Verification items for the finished model (mm, model axes). A direction names the side the tool comes from. Round coordinates to 2 decimals unless told otherwise and drop trailing zeros. Order: outer loops, then holes, each group sorted by start corner. A loop starts at its lowest first (then second) coordinate and runs counter-clockwise, first axis right, second up. Notation, with made-up numbers: (-29.75, 2.5) -> (28.25, 2.5) arc R15 ccw to (28.25, 19.5) -> close; hole circle Ø3 at (18.5, 4). An arc over 180 degrees is marked (long way). Put each result on its own line as item: value.
```python
from build123d import *
from build123d.topology import SkipClean

# Parameters (mm, degrees)
SKETCH1_R                = 20
SKETCH1_R_2              = 15
BOSS_EXTRUDE1_DEPTH      = 380
SKETCH8_R                = 20
BOSS_EXTRUDE3_DEPTH      = 60
CUT_EXTRUDE2_START       = -899.5
SKETCH9_R                = 15
CUT_EXTRUDE2_DEPTH       = 899.5
CUT_EXTRUDE16_DEPTH      = 240
CUT_EXTRUDE17_DEPTH      = 20
CUT_EXTRUDE17_DEPTH_BACK = 20
CUT_EXTRUDE19_DEPTH      = 10
CUT_EXTRUDE19_DEPTH_BACK = 10
SKETCH26_R               = 10
CUT_EXTRUDE20_DEPTH      = 30
CUT_EXTRUDE20_DEPTH_BACK = 20
SKETCH27_R               = 3.4


with BuildPart() as part:
    # Sketch1 → Boss-Extrude1 (new, symmetric)
    with BuildSketch(Plane(origin=(0, 0, 0), x_dir=(1, 0, 0), z_dir=(0, 1, 0))):
        with Locations(Location((0, 0, 0), (0, 0, 270))):
            Circle(SKETCH1_R)
        with Locations(Location((0, 0, 0), (0, 0, 270))):
            Circle(SKETCH1_R_2, mode=Mode.SUBTRACT)
    extrude(amount=BOSS_EXTRUDE1_DEPTH, both=True)

    # Sketch8 → Boss-Extrude3 (add)
    with SkipClean():  # the faces are left unmerged after this step: merging them gives an invalid solid
        with BuildSketch(Plane.XZ.offset(380)):
            with Locations(Location((0, 0, 0), (0, 0, 270))):
                Circle(SKETCH8_R)
        extrude(amount=BOSS_EXTRUDE3_DEPTH)

    # Sketch9 → Cut-Extrude2 (cut)
    with SkipClean():  # the faces are left unmerged after this step: merging them gives an invalid solid
        with BuildSketch(Plane(origin=(-32.302786122, 416.289190775, -45.221901395), x_dir=(-0.9768887275019512, 0, 0.2137484832217963), z_dir=(0, 1, 0)).offset(CUT_EXTRUDE2_START)):
            with Locations(Location((-21.890114798, 51.081437247, 0), (0, 0, 257.657886074))):
                Circle(SKETCH9_R)
        extrude(amount=CUT_EXTRUDE2_DEPTH, mode=Mode.SUBTRACT)

    # Sketch23 → Cut-Extrude16 (cut)
    with SkipClean():  # the faces are left unmerged after this step: merging them gives an invalid solid
        with BuildSketch(Plane(origin=(0, 380, 0), x_dir=(1, 0, 0), z_dir=(0, 1, 0))):
            with BuildLine():
                Line((-7, 18.734993995), (7, 18.734993995))
                ThreePointArc((7, 18.734993995), (0, 20), (-7, 18.734993995))
            make_face()
        cut_extrude16 = extrude(amount=-CUT_EXTRUDE16_DEPTH, mode=Mode.SUBTRACT)

    # Mirror1: Cut-Extrude16 across plane
    with SkipClean():  # the faces are left unmerged after this step: merging them gives an invalid solid
        add(cut_extrude16.mirror(Plane.XY), mode=Mode.SUBTRACT)

    # Sketch24 → Cut-Extrude17 (cut, two sides: drawn at the far end of the back side and taken through both)
    with SkipClean():  # the faces are left unmerged after this step: merging them gives an invalid solid
        with BuildSketch(Plane(origin=(0, 0, 0), x_dir=(0, 0, -1), z_dir=(1, 0, 0)).offset(-CUT_EXTRUDE17_DEPTH_BACK)):
            with BuildLine():
                Line((-0.5, 200), (0.5, 200))
                ThreePointArc((0.5, 200), (2.621320344, 199.121320344), (3.5, 197))
                Line((3.5, 197), (3.5, 9))
                ThreePointArc((3.5, 9), (2.621320344, 6.878679656), (0.5, 6))
                Line((0.5, 6), (-0.5, 6))
                ThreePointArc((-0.5, 6), (-2.621320344, 6.878679656), (-3.5, 9))
                Line((-3.5, 9), (-3.5, 197))
                ThreePointArc((-3.5, 197), (-2.621320344, 199.121320344), (-0.5, 200))
            make_face()
        extrude(amount=CUT_EXTRUDE17_DEPTH + CUT_EXTRUDE17_DEPTH_BACK, mode=Mode.SUBTRACT)

    # Sketch26 → Cut-Extrude19 (cut, two sides: drawn at the far end of the back side and taken through both)
    with SkipClean():  # the faces are left unmerged after this step: merging them gives an invalid solid
        with BuildSketch(Plane(origin=(0, -44.33037899, 18.734993995), x_dir=(1, 0, 0), z_dir=(0, 0, 1)).offset(-CUT_EXTRUDE19_DEPTH_BACK)):
            with Locations(Location((0, -101.15698714, 0), (0, 0, 180))):
                Circle(SKETCH26_R)
        extrude(amount=CUT_EXTRUDE19_DEPTH + CUT_EXTRUDE19_DEPTH_BACK, mode=Mode.SUBTRACT)

    # Sketch27 → Cut-Extrude20 (cut, two sides: drawn at the far end of the back side and taken through both)
    with SkipClean():  # the faces are left unmerged after this step: merging them gives an invalid solid
        with BuildSketch(Plane(origin=(0, -44.33037899, -18.734993995), x_dir=(-1, 0, 0), z_dir=(0, 0, -1)).offset(-CUT_EXTRUDE20_DEPTH_BACK)):
            with Locations(Location((0, -273.66962101, 0), (0, 0, 270))):
                Circle(SKETCH27_R)
            with Locations(Location((0, -288.66962101, 0), (0, 0, 270))):
                Circle(SKETCH27_R)
        extrude(amount=CUT_EXTRUDE20_DEPTH + CUT_EXTRUDE20_DEPTH_BACK, mode=Mode.SUBTRACT)


solid = part.part
```
Item 1: Depth check by flat-ended pin: pin 1 Ø15.5 at (x, y) = (-0.5, 315) entering from +Z (3 decimals); pin 2 Ø5.5 at (x, y) = (-17, 118.5) entering from +Z; pin 3 Ø1 at (y, z) = (58, -12) entering from +X. Enter the tip coordinate at first touch or a pass-through.
Geometry check:
pin 1: z = 18.735
pin 2: z = 14.03
pin 3: x = 16.36
Item 2: Release check for a two-part mould opening along Y. For faces 1 (the face through (9, 380, -13)), 2 (the face through (-9.54, -148.49, 15.53)), 3 (the face through (0, 262, 18.735)) record: pulls with the +Y half, pulls with the -Y half, needs draft (parallel to the pull), parting line crosses it, or undercut.
Geometry check:
face 1: pulls with the +Y half
face 2: undercut
face 3: needs draft
Item 3: Sectioned sample at A-A, the plane y = 151.5. Record the boundary of the cut face in (x, z) (3 decimals).
Geometry check:
outline: (-19.691, -3.5) arc R20 ccw to (-7, -18.735) -> (7, -18.735) arc R20 ccw to (19.691, -3.5) -> (14.586, -3.5) arc R15 cw to (-14.586, -3.5) -> close; (-19.691, 3.5) -> (-14.586, 3.5) arc R15 cw to (14.586, 3.5) -> (19.691, 3.5) arc R20 ccw to (7, 18.735) -> (-7, 18.735) arc R20 ccw to start
Item 4: Material ranges on line 1 along X through (y, z) = (-136.5, 0.5); line 2 along Y through (x, z) = (17, 0); line 3 along Z through (x, y) = (1.5, -220), recorded low to high.
Geometry check:
line 1: -19.99 to -14.99, 14.99 to 19.99
line 2: -440 to 6, 200 to 380
line 3: -19.94 to -14.92, 14.92 to 19.94
Item 5: Tool access check on faces 4 (the face through (0, 262, -18.735)), 5 (the face through (15, -440, -3)). Record the directions out of +Z, -Z, +X, -X, +Y, -Y that give a thin tool (end or side, any length) a straight path to the whole face; none if there is none.
Geometry check:
face 4: -Z, +X, -X, +Y
face 5: +Z, -Z, +X, -X, -Y
Item 6: Sectioned sample at B-B, the plane y = -24.5. Record the boundary of the cut face in (x, z), then the cut area to 3 significant figures.
Geometry check:
outline: circle Ø40 at (0, 0); hole circle Ø30 at (0, 0)
area: 550 mm2
